For this review, take the finished solid that the model builds, in its own axes (mm). Face numbers are marked on the shaded views. A direction names the side the tool comes from. Coordinates: 2 decimals unless noted, no trailing zeros. Order: outer loops, then holes, each group sorted by start corner. A loop starts at its lowest first (then second) coordinate and runs counter-clockwise, first axis right, second up.
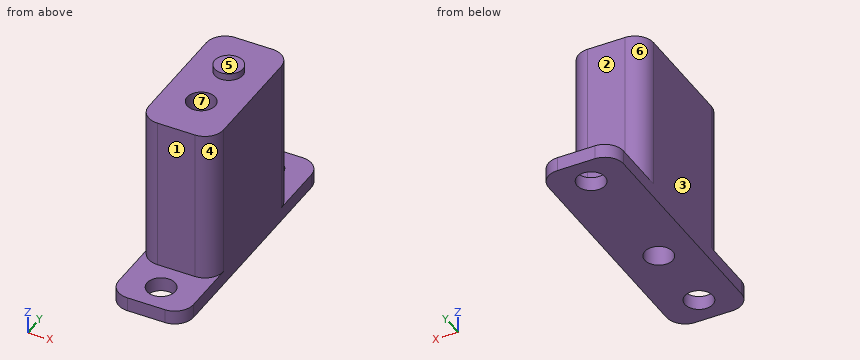
from build123d import *

# Parameters (mm, degrees)
F0_W     = 8
F0_H     = 15.5
F0_R     = 1.5
F1_DEPTH = 18
F2_D     = 3
F3_DEPTH = 0.75
F4_W     = 8
F4_H     = 6
F5_DEPTH = 1.5
F6_D     = 3
F7_R     = 2


with BuildPart() as f1:
    # F0 (on Top) → F1 (new body)
    with BuildSketch(Plane.XY):
        with Locations((4, 7.75)):
            Rectangle(F0_W, F0_H)
        with Locations((4, 10.5)):
            Circle(F0_R, mode=Mode.SUBTRACT)
        with Locations((4, 10.5)):
            Circle(F0_R)
    extrude(amount=-F1_DEPTH)

    # F2 (through all)
    with Locations(Plane.XY):
        with Locations((4, 5)):
            Hole(F2_D / 2)

    # F0 (on Top) → F3 (join)
    with BuildSketch(Plane.XY):
        with Locations((4, 10.5)):
            Circle(F0_R)
    extrude(amount=F3_DEPTH)

    # F4 (on face) → F5 (join)
    with BuildSketch(Plane(origin=(0, 0, -18), x_dir=(1, 0, 0), z_dir=(0, 0, -1))):
        with Locations((4, 3)):
            Rectangle(F4_W, F4_H)
        with Locations((4, -18.5)):
            Rectangle(F4_W, F4_H)
    extrude(amount=-F5_DEPTH)

    # F6 (through all)
    with Locations(Plane(origin=(0, 0, -18), x_dir=(1, 0, 0), z_dir=(0, 0, -1))):
        with Locations((4, 3), (4, -18.5)):
            Hole(F6_D / 2)

    # F7
    f7_edges = [f1.edges().sort_by_distance(p)[0] for p in [
        (0, 0, -8.25),
        (8, 0, -8.25),
        (8, 15.5, -8.25),
        (0, 15.5, -8.25),
        (8, -6, -17.25),
        (0, -6, -17.25),
        (8, 21.5, -17.25),
        (0, 21.5, -17.25),
    ]]
    fillet(f7_edges, radius=F7_R)


solid = f1.part
1. Take a section at C-C, the plane x = 4. Give the boundary of the cut face in (y, z).
Answer below:
outline: (-6, -18) - (-4.5, -18) - (-4.5, -16.5) - (-6, -16.5) - close; (-1.5, -18) - (3.5, -18) - (3.5, 0) - (0, 0) - (0, -16.5) - (-1.5, -16.5) - close; (6.5, -18) - (17, -18) - (17, -16.5) - (15.5, -16.5) - (15.5, 0) - (12, 0) - (12, 0.75) - (9, 0.75) - (9, 0) - (6.5, 0) - close; (20, -18) - (21.5, -18) - (21.5, -16.5) - (20, -16.5) - close
2. Take a section at B-B, the plane z = -4.5. Give the boundary of the cut face in (x, y), plus the area to 3 significant figures.
Answer below:
outline: (0, 2) arc R2 ccw to (2, 0) - (6, 0) arc R2 ccw to (8, 2) - (8, 13.5) arc R2 ccw to (6, 15.5) - (2, 15.5) arc R2 ccw to (0, 13.5) - close; hole circle Ø3 at (4, 5)
area: 113 mm2
3. Take a section at D-D, the plane y = 5. Give the boundary of the cut face in (x, z), plus the area to 3 significant figures.
Answer below:
outline: (0, -18) - (2.5, -18) - (2.5, 0) - (0, 0) - close; (5.5, -18) - (8, -18) - (8, 0) - (5.5, 0) - close
area: 90.0 mm2
4. Machinability: for the marked faces 1, 2, 3 and 4, which of the approach directions +Z, -Z, +X, -X, +Y, -Y give a long, thin tool a straight path to every point of the face, cutting with its end or side? Answer none if there is none.
Answer below:
face 1: +Z, +X, -X, -Y
face 2: +Z, +X, -X, +Y
face 3: +Z, -Z, -X, +Y, -Y
face 4: +Z, +X, -Y
5. The part is to be moulded in two halves that separate along X. For the marked faces 5, 6 and 7, say which applies: +X half, -X half, draft (parallel to the pull), parting line (faces both ways), or undercut.
Answer below:
face 5: draft
face 6: -X half
face 7: undercut
6. Take a section at A-A, the plane y = 18.5. Give the boundary of the cut face in (x, z), plus the area to 3 significant figures.
Answer below:
outline: (0, -18) - (2.5, -18) - (2.5, -16.5) - (0, -16.5) - close; (5.5, -18) - (8, -18) - (8, -16.5) - (5.5, -16.5) - close
area: 7.50 mm2
7. To check wall thickness, follow L1, parallel to Y at x = 4, z = -17.6; L2, parallel to Y at x = 4, z = -9.5; L3, parallel to X at y = 18.5, z = -17.1. State the ranges of each line that lie inside material, in increasing order.
Answer below:
L1: y = -6 to -4.5, -1.5 to 3.5, 6.5 to 17, 20 to 21.5
L2: y = 0 to 3.5, 6.5 to 15.5
L3: x = 0 to 2.5, 5.5 to 8
8. Clearance check with flat-ended pins moving along their axes: pin 1 Ø2 at (x, z) = (4.5, -5) entering from -Y; pin 2 Ø1.8 at (x, y) = (4, 18.5) entering from +Z; pin 3 Ø4.5 at (x, z) = (3.5, -9.5) entering from +Y; pin 4 Ø2.5 at (x, y) = (4, -2) entering from +Z. State where each tip first meets the part, or that it passes through.
Answer below:
pin 1: stops at y = 0
pin 2: passes through
pin 3: stops at y = 15.5
pin 4: stops at z = -16.5
